Design review of the part built by this model. Coordinates are the model's own, in mm. A direction names the side the tool comes from. Coordinates: 2 decimals unless noted, no trailing zeros. Write each loop counter-clockwise with the first axis right and the second up, starting at its lowest first coordinate (ties: lowest second). Pieces come first, ordered by that corner, then holes.
Q1. Take a section at D-D (x = 20.5). Give the boundary of the cut face in (y, z).
Q2. For probe 1 along Y at (x, z) = (-36.83, 3) (3 decimals); probe 2 along Y at (x, z) = (-11.5, 3.25); probe 3 along X at (y, z) = (-11.5, 5.25), list the stretches that pass through material, from the lowest coordinate up.
Q3. Mouldability with a two-part tool opening along X and no side actions: class faces 1 (the cylindrical face through (-49.53, 0.39, 3.13)), 2 (the flat face through (-37.672, -26.395, 3.131)), 3 (the flat face through (0, 0, 0)) as pulls with the +X half, pulls with the -X half, needs draft (parallel to the pull), parting line crosses it, or undercut.
Q4. Insertion check: pin 1 (1.5 mm diameter, centred on y = 18.5, z = 4.5, fed in from -X). The pin has a flat end and moves straight along its axis. Give the tip position at first contact, or say it passes through.
Q5. Take a section at A-A (y = 0). Give the boundary of the cut face in (x, z) (3 decimals), and give its area (3 significant figures).
Q6. Take a section at B-B (z = 1). Give the boundary of the cut face in (x, y) (3 decimals), and give its area (3 significant figures).
Q7. Machinability: for faces 4 (the flat face through (0, -5.08, 3)), 5 (the cylindrical face through (36.88, -12.07, 3.22)), 6 (the flat face through (37.72, 26.43, 3.13)), which of the approach directions +Z, -Z, +X, -X, +Y, -Y give a long, thin tool a straight path to every point of the face, cutting with its end or side? Answer none if there is none.
Q8. Take a section at C-C (y = 24). Give the boundary of the cut face in (x, z).
```python
from build123d import *

# Parameters (mm, degrees)
SKETCH1_R           = 49.53
BOSS_EXTRUDE2_DEPTH = 6.35
FILLET2_R           = 12.7
FILLET3_R           = 12.7
FILLET4_R           = 12.7
FILLET5_R           = 12.7
CUT_EXTRUDE1_DEPTH  = 6.35
SKETCH3_R           = 3.175
CUT_EXTRUDE2_DEPTH  = 6.35
FILLET6_R           = 1.27
FILLET7_R           = 1.27
FILLET8_R           = 1.27
FILLET9_R           = 1.27


with BuildPart() as part:
    # Sketch1 → Boss-Extrude2 (new body)
    with BuildSketch(Plane.XY):
        Circle(SKETCH1_R)
        with BuildLine():
            Line((-43.519510854, 5.08), (43.519510854, 5.08))
            ThreePointArc((43.519510854, 5.08), (0, 43.815), (-43.519510854, 5.08))
        make_face(mode=Mode.SUBTRACT)
        with BuildLine():
            Line((-43.519510854, -5.08), (43.519510854, -5.08))
            ThreePointArc((43.519510854, -5.08), (0, -43.815), (-43.519510854, -5.08))
        make_face(mode=Mode.SUBTRACT)
    extrude(amount=BOSS_EXTRUDE2_DEPTH)

    # Fillet2
    fillet2_edges = [part.edges().sort_by_distance(p)[0] for p in [
        (43.519510854, 5.08, 3.175),
    ]]
    fillet(fillet2_edges, radius=FILLET2_R)

    # Fillet3
    fillet3_edges = [part.edges().sort_by_distance(p)[0] for p in [
        (-43.519510854, 5.08, 3.175),
    ]]
    fillet(fillet3_edges, radius=FILLET3_R)

    # Fillet4
    fillet4_edges = [part.edges().sort_by_distance(p)[0] for p in [
        (43.519510854, -5.08, 3.175),
    ]]
    fillet(fillet4_edges, radius=FILLET4_R)

    # Fillet5
    fillet5_edges = [part.edges().sort_by_distance(p)[0] for p in [
        (-43.519510854, -5.08, 3.175),
    ]]
    fillet(fillet5_edges, radius=FILLET5_R)

    # Sketch2 → Cut-Extrude1 (cut)
    with BuildSketch(Plane(origin=(0, 0, 0), x_dir=(-1, 0, 0), z_dir=(0, 0, -1))):
        with BuildLine():
            Line((-40.581029215, -28.3972), (-35.898602767, -25.1206))
            ThreePointArc((-35.898602767, -25.1206), (-0.013001801, -43.814998071), (35.883687713, -25.141900904))
            Line((35.883687713, -25.141900904), (40.564168719, -28.421279283))
            ThreePointArc((40.564168719, -28.421279283), (-0.014697689, -49.529997819), (-40.581029215, -28.3972))
        make_face()
        with BuildLine():
            Line((-40.564168719, 28.421279283), (-35.883687713, 25.141900904))
            ThreePointArc((-35.883687713, 25.141900904), (0.013001801, 43.814998071), (35.898602767, 25.1206))
            Line((35.898602767, 25.1206), (40.581029215, 28.3972))
            ThreePointArc((40.581029215, 28.3972), (0.014697689, 49.529997819), (-40.564168719, 28.421279283))
        make_face()
    extrude(amount=-CUT_EXTRUDE1_DEPTH, mode=Mode.SUBTRACT)

    # Sketch3 → Cut-Extrude2 (cut)
    with BuildSketch(Plane(origin=(0, 0, 0), x_dir=(-1, 0, 0), z_dir=(0, 0, -1))):
        with Locations((-36.83, 0)):
            Circle(SKETCH3_R)
        with Locations(Location((36.83, 0, 0), (0, 0, 180))):
            Circle(SKETCH3_R)
    extrude(amount=-CUT_EXTRUDE2_DEPTH, mode=Mode.SUBTRACT)

    # Fillet6
    fillet6_edges = [part.edges().sort_by_distance(p)[0] for p in [
        (-40.581029215, 28.3972, 3.175),
    ]]
    fillet(fillet6_edges, radius=FILLET6_R)

    # Fillet7
    fillet7_edges = [part.edges().sort_by_distance(p)[0] for p in [
        (-40.564168719, -28.421279283, 3.175),
    ]]
    fillet(fillet7_edges, radius=FILLET7_R)

    # Fillet8
    fillet8_edges = [part.edges().sort_by_distance(p)[0] for p in [
        (40.581029215, -28.3972, 3.175),
    ]]
    fillet(fillet8_edges, radius=FILLET8_R)

    # Fillet9
    fillet9_edges = [part.edges().sort_by_distance(p)[0] for p in [
        (40.564168719, 28.421279283, 3.175),
    ]]
    fillet(fillet9_edges, radius=FILLET9_R)


solid = part.part
```
Response:
1. outline: (-5.08, 0) - (5.08, 0) - (5.08, 6.35) - (-5.08, 6.35) - close
2. probe 1: y = -25.805 to -23.585, -11.975 to -3.175, 3.175 to 11.975, 23.585 to 25.772
2. probe 2: y = -5.08 to 5.08
2. probe 3: x = -48.18 to -36.57, 36.57 to 48.18
3. face 1: pulls with the -X half
3. face 2: undercut
3. face 3: needs draft
4. pin 1: stops at x = -46.24
5. outline: (-49.53, 0) - (-40.005, 0) - (-40.005, 6.35) - (-49.53, 6.35) - close; (-33.655, 0) - (33.655, 0) - (33.655, 6.35) - (-33.655, 6.35) - close; (40.005, 0) - (49.53, 0) - (49.53, 6.35) - (40.005, 6.35) - close
5. area: 548 mm2
6. outline: (-41.314, 27.319) arc R49.53 ccw to (-41.298, -27.344) arc R1.27 ccw to (-39.51, -27.683) - (-35.884, -25.142) arc R43.815 cw to (-35.957, -25.037) arc R12.7 cw to (-25.535, -5.08) - (25.535, -5.08) arc R12.7 cw to (35.957, -25.037) arc R43.815 cw to (35.899, -25.121) - (39.527, -27.659) arc R1.27 ccw to (41.314, -27.319) arc R49.53 ccw to (41.298, 27.344) arc R1.27 ccw to (39.51, 27.683) - (35.884, 25.142) arc R43.815 cw to (35.957, 25.037) arc R12.7 cw to (25.535, 5.08) - (-25.535, 5.08) arc R12.7 cw to (-35.957, 25.037) arc R43.815 cw to (-35.899, 25.121) - (-39.527, 27.659) arc R1.27 ccw to start; hole circle Ø6.35 at (-36.83, 0); hole circle Ø6.35 at (36.83, 0)
6. area: 1,830 mm2
7. face 4: +Z, -Z, -Y
7. face 5: +Z, -Z
7. face 6: +Z, -Z, +Y
8. outline: (-43.33, 0) - (-36.61, 0) - (-36.61, 6.35) - (-43.33, 6.35) - close; (36.61, 0) - (43.33, 0) - (43.33, 6.35) - (36.61, 6.35) - close
